from build123d import *

# Parameters (mm, degrees)
F1_W        = 33.513052389
F1_H        = 43.4953216463
F2_DEPTH    = 25
F0_W        = 27.636364032
F0_H        = 36
F3_DEPTH    = 25
F4_W        = 33.513052389
F4_H        = 36
F5_DEPTH    = 20
F6_T1_DEPTH = 58.1822545614
F6_T3_DEPTH = 57.0345340949
F7_W        = 34
F7_H        = 90
F8_DEPTH    = 4
F9_T1_DEPTH = 58.4948974279
F10_R       = 5
F11_DEPTH   = 0.5


# Not quite as in the source:
# - a fillet or chamfer that OpenCascade refuses, or shapes differently, is made with other operations: its cross-section is extruded or revolved along the edge and cut away or added


with BuildPart() as f2:
    # F1 (on Top) → F2 (new body)
    with BuildSketch(Plane.XY):
        with Locations((-35.7246743515, 1.4273980632)):
            Rectangle(F1_W, F1_H)
    extrude(amount=F2_DEPTH)

    # F0 (on Top) → F3 (cut)
    with BuildSketch(Plane.XY):
        with Locations((-35.9798576683, 0.9857490659)):
            Rectangle(F0_W, F0_H)
    extrude(amount=F3_DEPTH, mode=Mode.SUBTRACT)

    # F4 (on face) → F5 (cut)
    with BuildSketch(Plane.XY.offset(25)):
        with Locations((-35.7246743515, 0.9857490659)):
            Rectangle(F4_W, F4_H)
    extrude(amount=-F5_DEPTH, mode=Mode.SUBTRACT)

    # F6: fillet of radius 5 on 2 edges, made by hand

    # F6_s2 → F6_t1 (cut)
    with BuildSketch(Plane.YZ.offset(-64.8158016322)):
        with BuildLine():
            ThreePointArc((23.1750588864, 20.0661595655), (21.9864530472, 23.302403461), (18.9857490659, 25))
            Line((18.9857490659, 25), (23.1750588864, 25))
            Line((23.1750588864, 25), (23.1750588864, 20.0661595655))
        make_face()
    extrude(amount=F6_T1_DEPTH, mode=Mode.SUBTRACT)

    # F6_s4 → F6_t3 (cut)
    with BuildSketch(Plane.YZ.offset(-64.241941399)):
        with BuildLine():
            ThreePointArc((-17.0142509341, 25), (-19.4111025802, 23.170600103), (-20.3202627599, 20.2957036588))
            Line((-20.3202627599, 20.2957036588), (-20.3202627599, 25))
            Line((-20.3202627599, 25), (-17.0142509341, 25))
        make_face()
    extrude(amount=F6_T3_DEPTH, mode=Mode.SUBTRACT)

    # F7 (on Top) → F8 (join)
    with BuildSketch(Plane.XY):
        with Locations((-35.3662480154, -0.4606725276)):
            Rectangle(F7_W, F7_H)
    extrude(amount=F8_DEPTH)

    # F9: fillet of radius 5 on 2 edges, made by hand

    # F9_s2 → F9_t1 (cut)
    with BuildSketch(Plane.YZ.offset(-64.6136967294)):
        with BuildLine():
            ThreePointArc((-40.561693042, 4), (-43.7239707021, 2.8729833462), (-45.4606725275, 0))
            Line((-45.4606725275, 0), (-45.4606725276, 4))
            Line((-45.4606725276, 4), (-40.561693042, 4))
        make_face()
        with BuildLine():
            ThreePointArc((39.6403479869, 4), (42.802625647, 2.8729833462), (44.5393274724, 0))
            Line((44.5393274724, 0), (44.5393274724, 4))
            Line((44.5393274724, 4), (39.6403479869, 4))
        make_face()
    extrude(amount=F9_T1_DEPTH, mode=Mode.SUBTRACT)

    # F10
    f10_edges = [f2.edges().sort_by_distance(p)[0] for p in [
        (-35.667198, -20.320263, 4),
        (-35.667198, 23.175059, 4),
    ]]
    fillet(f10_edges, radius=F10_R)

    # F11 (cut): a face of the model
    f11_faces = [f2.faces().sort_by_distance(p)[0] for p in [
        (-18.3662480154, -0.4606725276, 1.9725049158),
    ]]
    extrude(f11_faces, amount=-F11_DEPTH, mode=Mode.SUBTRACT)


solid = f2.part
Part model, mm, in its own coordinate system. A direction names the side the tool comes from. Round coordinates to 2 decimals unless told otherwise and drop trailing zeros. Loops run counter-clockwise (first coordinate to the right, second up) from the corner with the lowest first, then second, coordinate; pieces in that order, holes last. Notation, with made-up numbers: (61.5, 28.25) - (90.5, 28.25) arc R6 cw to (90.5, 36.25) - close; hole circle Ø9 at (-22.75, -9). An arc over 180 degrees is marked (long way). Answer as a JSON object with one key per item and string values.
Item 1: Band-saw the part on C-C on x = -43.5. List the corners of the cut face in (y, z), plus the area to 3 significant figures.
Output:
{"outline": "(-45.46, 0) - (44.54, 0) arc R5 ccw to (39.64, 4) - (28.18, 4) arc R5 cw to (23.18, 9) - (23.18, 20.07) arc R5 ccw to (18.99, 25) - (18.99, 4) - (-17.01, 4) - (-17.01, 25) arc R5 ccw to (-20.32, 20.3) - (-20.32, 9) arc R5 cw to (-25.32, 4) - (-40.56, 4) arc R5 ccw to start", "area": "509 mm2"}
Item 2: Tool access for faces 1 (the face through (-21, 1, 5)), 2 (the face through (-52.366, -33, 2)), 3 (the face through (-18.968, 7.2, 4.3)), 4 (the face through (-52.366, 34, 2)), 5 (the face through (-35.96, 22.02, 23.26)): list every direction of +Z, -Z, +X, -X, +Y, -Y with a clear straight run to the whole face (end or side of a thin tool).
Output:
{"face 1": "+Z, +X, -X", "face 2": "+Z, -Z, -X, -Y", "face 3": "+Z, +X, +Y, -Y", "face 4": "+Z, -Z, -X, +Y", "face 5": "+Z, +X, -X, +Y"}
Item 3: Band-saw the part on B-B on y = -9. List the corners of the cut face in (x, z), plus the area to 3 significant figures.
Output:
{"outline": "(-52.48, 0) - (-18.87, 0) - (-18.87, 4) - (-18.97, 4) - (-18.97, 5) - (-22.16, 5) - (-22.16, 4) - (-49.8, 4) - (-49.8, 5) - (-52.48, 5) - close", "area": "140 mm2"}
Item 4: Band-saw the part on D-D on z = 2.25. List the corners of the cut face in (x, y), plus the area to 3 significant figures.
Output:
{"outline": "(-52.48, -20.32) - (-52.37, -20.32) - (-52.37, -44.36) - (-18.87, -44.36) - (-18.87, 43.44) - (-52.37, 43.44) - (-52.37, 23.18) - (-52.48, 23.18) - close", "area": "2,950 mm2"}
Item 5: Wall check: L1, parallel to Y at x = -46, z = 11.5; L2, parallel to X at y = -40.5, z = 3.5; L3, parallel to Z at x = -37, y = -35.5. Give the ranges that are in metal, low to high.
Output:
{"L1": "-20.32 to -17.01, 18.99 to 23.18", "L2": "-52.37 to -18.87", "L3": "0 to 4"}
Item 6: Band-saw the part on A-A on z = 19.25. List the corners of the cut face in (x, y).
Output:
{"outline": "(-52.48, -20.32) - (-18.97, -20.32) - (-18.97, -17.01) - (-52.48, -17.01) - close; (-52.48, 18.99) - (-18.97, 18.99) - (-18.97, 23.18) - (-52.48, 23.18) - close"}
Item 7: Pin check, flat tips, straight feed: pin 1 (1.3 mm diameter, centred on x = -51, y = 5, fed in from +Z); pin 2 (4.5 mm diameter, centred on y = -35, z = 5.5, fed in from -X); pin 3 (1.5 mm diameter, centred on x = -36.5, z = 5.5, fed in from -Y); pin 4 (2 mm diameter, centred on x = -26.5, y = -32.5, fed in from -Z). Stop position of each tip, or through.
Output:
{"pin 1": "z = 5", "pin 2": "x = -52.37", "pin 3": "y = -22.69", "pin 4": "z = 0"}
Item 8: Pull direction Y, two halves, no side cores. Call faces 6 (the face through (-36, 1, 4)), 7 (the face through (-36, 18.986, 15)), 8 (the face through (-35.959, -19.386, 23.206)), 9 (the face through (-18.866, -1, 2)): pulls with the +Y half, pulls with the -Y half, needs draft (parallel to the pull), parting line crosses it, or undercut.
Output:
{"face 6": "undercut", "face 7": "undercut", "face 8": "pulls with the -Y half", "face 9": "needs draft"}
